from build123d import *

# Parameters (mm, degrees)
SKETCH1_R           = 20.5
SKETCH1_R_2         = 3
SKETCH1_W           = 17
SKETCH1_H           = 14
BOSS_EXTRUDE1_DEPTH = 3
FILLET1_R           = 2


with BuildPart() as part:
    # Sketch1 → Boss-Extrude1 (new body)
    with BuildSketch(Plane.XY):
        Circle(SKETCH1_R)
        with Locations((-13, 0)):
            Circle(SKETCH1_R_2, mode=Mode.SUBTRACT)
        with Locations((13, 0)):
            Circle(SKETCH1_R_2, mode=Mode.SUBTRACT)
        Rectangle(SKETCH1_W, SKETCH1_H, mode=Mode.SUBTRACT)
    extrude(amount=BOSS_EXTRUDE1_DEPTH)

    # Fillet1
    fillet1_edges = [part.edges().sort_by_distance(p)[0] for p in [
        (8.5, -7, 1.5),
        (8.5, 7, 1.5),
        (-8.5, 7, 1.5),
        (-8.5, -7, 1.5),
    ]]
    fillet(fillet1_edges, radius=FILLET1_R)


solid = part.part
Could you check a few things on this model? Use its own coordinates, in mm. A direction names the side the tool comes from. Coordinates: 2 decimals unless noted, no trailing zeros. Loops run counter-clockwise (first coordinate to the right, second up) from the corner with the lowest first, then second, coordinate; pieces in that order, holes last.
1. I need wall thicknesses on L1, parallel to X at y = 0.5, z = 2; L2, parallel to X at y = -2.5, z = 1.6; L3, parallel to Y at x = -0.5, z = 1.25. Which ranges of each line are inside material? Lowest first, please.
2. Imagine slicing it at C-C (x = -3.5). Please give me the cut outline in (y, z).
3. For P1, Ø1, axis at x = 12, z = 1, coming from the +Y side; P2, Ø0.9, axis at x = 2, z = 1.5, coming from the -Y side, each with a flat end and sliding along its axis, tell me the tip position at first contact or that it passes through.
4. Imagine slicing it at A-A (y = 0). Please give me the cut outline in (x, z), and give its area (3 significant figures).
5. We'd pull the mould along X, two halves only. Please class faces 3 (the face through (-7.9, -6.43, 1.52)), 4 (the face through (-4.444, -20.013, 1.479)), 5 (the face through (0, -9, 0)): released by +X, released by -X, zero draft, split by the parting line, or undercut.
6. Imagine slicing it at D-D (y = 6.5). Please give me the cut outline in (x, z).
7. For faces 1 (the face through (0, -9, 3)), 2 (the face through (-8.5, 0, 1)), which set-ups out of +Z, -Z, +X, -X, +Y, -Y let a thin tool reach every point of the face, with its end or its side?
8. Imagine slicing it at B-B (z = 0.45). Please give me the cut outline in (x, y), and give its area (3 significant figures).
Computed values:
1. L1: x = -20.49 to -15.96, -10.04 to -8.5, 8.5 to 10.04, 15.96 to 20.49
1. L2: x = -20.35 to -14.66, -11.34 to -8.5, 8.5 to 11.34, 14.66 to 20.35
1. L3: y = -20.49 to -7, 7 to 20.49
2. outline: (-20.2, 0) - (-7, 0) - (-7, 3) - (-20.2, 3) - close; (7, 0) - (20.2, 0) - (20.2, 3) - (7, 3) - close
3. P1: stops at y = 16.97
3. P2: stops at y = -20.44
4. outline: (-20.5, 0) - (-16, 0) - (-16, 3) - (-20.5, 3) - close; (-10, 0) - (-8.5, 0) - (-8.5, 3) - (-10, 3) - close; (8.5, 0) - (10, 0) - (10, 3) - (8.5, 3) - close; (16, 0) - (20.5, 0) - (20.5, 3) - (16, 3) - close
4. area: 36.0 mm2
5. face 3: undercut
5. face 4: split by the parting line
5. face 5: zero draft
6. outline: (-19.44, 0) - (-7.82, 0) - (-7.82, 3) - (-19.44, 3) - close; (7.82, 0) - (19.44, 0) - (19.44, 3) - (7.82, 3) - close
7. face 1: +Z, +X, -X, +Y, -Y
7. face 2: +Z, -Z
8. outline: circle Ø41 at (0, 0); hole circle Ø6 at (-13, 0); hole (-8.5, -5) arc R2 ccw to (-6.5, -7) - (6.5, -7) arc R2 ccw to (8.5, -5) - (8.5, 5) arc R2 ccw to (6.5, 7) - (-6.5, 7) arc R2 ccw to (-8.5, 5) - close; hole circle Ø6 at (13, 0)
8. area: 1,030 mm2
